Study the drawing (mm; zero at the part's minimum x, y, z) and answer. A direction names the side the tool comes from. Coordinates: 2 decimals unless noted, no trailing zeros. Write each loop counter-clockwise with the first axis right and the second up, starting at its lowest first coordinate (ties: lowest second). Pieces come first, ordered by that corner, then holes. Notation, with made-up numbers: (58, 89.25) - (102, 89.25) arc R19 cw to (102, 107.25) - close; hole circle Ø4 at (42.25, -11.75). An arc over 180 degrees is marked (long way). One line per item, written item: value.
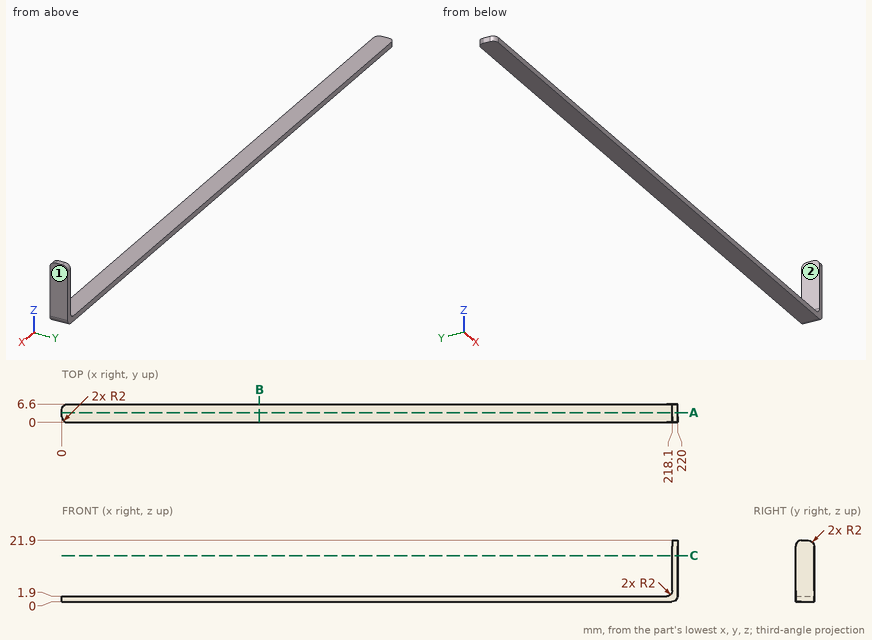
Item 1: Consider probe 1 along Z at (x, y) = (12.5, 5); probe 2 along X at (y, z) = (1, 20.5); probe 3 along X at (y, z) = (3, 1.75). Determine where each line is inside the solid, lowest interval first.
Evaluation:
probe 1: z = 0 to 1.9
probe 2: x = 218.1 to 220
probe 3: x = 0 to 219.98
Item 2: Section A-A, the plane y = 3.5 is taken. Determine the outline of the cut face in (x, z).
Evaluation:
outline: (0, 0) - (218, 0) arc R2 ccw to (220, 2) - (220, 21.9) - (218.1, 21.9) - (218.1, 3.9) arc R2 cw to (216.1, 1.9) - (0, 1.9) - close
Item 3: Section B-B, the plane x = 70.5 is taken. Determine the outline of the cut face in (y, z), then the cut area to 3 significant figures.
Evaluation:
outline: (0, 0) - (6.6, 0) - (6.6, 1.9) - (0, 1.9) - close
area: 12.5 mm2
Item 4: Given pin 1 (2 mm diameter, centred on x = 182, y = 3.5, fed in from +Z), flat-ended and moving along its own axis, determine where the tip first touches the part or whether it passes through.
Evaluation:
pin 1: stops at z = 1.9
Item 5: Which of the six approach directions +Z, -Z, +X, -X, +Y, -Y give full straight-line access (tool end or side, diameter ignored) to the marked faces 1 and 2?
Evaluation:
face 1: +Z, -Z, +X, +Y, -Y
face 2: +Z, -X, +Y, -Y
Item 6: Section C-C, the plane z = 16.5 is taken. Determine the outline of the cut face in (x, y).
Evaluation:
outline: (218.1, 0) - (220, 0) - (220, 6.6) - (218.1, 6.6) - close
